Can you work these out from the model? Positions are in its coordinate system, mm. Give positions to 0.01 mm unless a question says otherwise; leave off trailing zeros. Order: outer loops, then holes, each group sorted by start corner. A loop starts at its lowest first (then second) coordinate and runs counter-clockwise, first axis right, second up. Notation, with made-up numbers: (-29.75, 72) - (-24.75, 72) arc R8 ccw to (-24.75, 80) - close; hole circle Ø6 at (78.5, 69.5). An arc over 180 degrees is marked (long way). Answer as a JSON object with one key per item and string values.
```python
from build123d import *

# Parameters (mm, degrees)
BOSS_EXTRUDE1_DEPTH  = 4.7625
M4_CLEARANCE_HOLE1_D = 4.5


with BuildPart() as part:
    # Sketch2 → Boss-Extrude1 (new body)
    with BuildSketch(Plane.XY):
        with BuildLine():
            Line((-58.18125, 21.734258268), (-58.18125, -30.061313165))
            ThreePointArc((-58.18125, -30.061313165), (-59.147979937, -34.921392756), (-61.900993879, -39.041569286))
            Line((-61.900993879, -39.041569286), (-63.182817689, -40.323393096))
            ThreePointArc((-63.182817689, -40.323393096), (-63.182817689, -48.101567689), (-55.404643096, -48.101567689))
            Line((-55.404643096, -48.101567689), (-54.122819286, -46.819743879))
            ThreePointArc((-54.122819286, -46.819743879), (-50.002642756, -44.066729937), (-45.142563165, -43.1))
            Line((-45.142563165, -43.1), (45.142563165, -43.1))
            ThreePointArc((45.142563165, -43.1), (50.002642756, -44.066729937), (54.122819286, -46.819743879))
            Line((54.122819286, -46.819743879), (55.404643096, -48.101567689))
            ThreePointArc((55.404643096, -48.101567689), (63.182817689, -48.101567689), (63.182817689, -40.323393096))
            Line((63.182817689, -40.323393096), (61.900993879, -39.041569286))
            ThreePointArc((61.900993879, -39.041569286), (59.147979937, -34.921392756), (58.18125, -30.061313165))
            Line((58.18125, -30.061313165), (58.18125, 21.734258268))
            ThreePointArc((58.18125, 21.734258268), (59.919591901, 28.147685724), (64.658738462, 32.805407718))
            ThreePointArc((64.658738462, 32.805407718), (67.284676339, 38.9927926), (61.96395, 43.1))
            Line((61.96395, 43.1), (-61.96395, 43.1))
            ThreePointArc((-61.96395, 43.1), (-67.284676339, 38.9927926), (-64.658738462, 32.805407718))
            ThreePointArc((-64.658738462, 32.805407718), (-59.919591901, 28.147685724), (-58.18125, 21.734258268))
        make_face()
    extrude(amount=BOSS_EXTRUDE1_DEPTH)

    # M4 Clearance Hole1 (through all)
    with Locations(Plane.XY.offset(4.7625)):
        with Locations((-59.293730392, -44.212480392), (-61.96395, 37.6), (61.96395, 37.6), (59.293730392, -44.212480392)):
            Hole(M4_CLEARANCE_HOLE1_D / 2)


solid = part.part
```
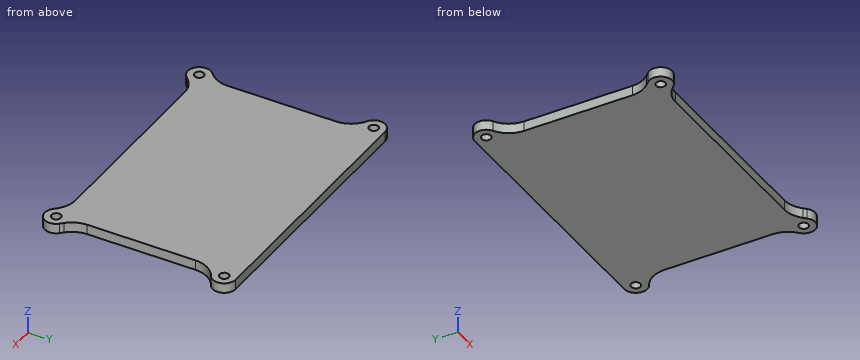
Q1. If we section it at A-A, the plane y = 37.6: Please give me the cut outline in (x, z).
Recorded:
{"outline": "(-67.46, 0) - (-64.21, 0) - (-64.21, 4.76) - (-67.46, 4.76) - close; (-59.71, 0) - (59.71, 0) - (59.71, 4.76) - (-59.71, 4.76) - close; (64.21, 0) - (67.46, 0) - (67.46, 4.76) - (64.21, 4.76) - close"}
Q2. I need wall thicknesses on L1, parallel to X at y = -10, z = 3.1; L2, parallel to Y at x = 37.5, z = 1.45; L3, parallel to Y at x = 58, z = 4.2. Which ranges of each line are inside material? Lowest first, please.
Recorded:
{"L1": "x = -58.18 to 58.18", "L2": "y = -43.1 to 43.1", "L3": "y = -49.56 to -46.05, -42.37 to 43.1"}
Q3. If we section it at C-C, the plane z = 3.1: Please give me the cut outline in (x, y).
Recorded:
{"outline": "(-64.66, 32.81) arc R12.7 cw to (-58.18, 21.73) - (-58.18, -30.06) arc R12.7 cw to (-61.9, -39.04) - (-63.18, -40.32) arc R5.5 ccw to (-55.4, -48.1) - (-54.12, -46.82) arc R12.7 cw to (-45.14, -43.1) - (45.14, -43.1) arc R12.7 cw to (54.12, -46.82) - (55.4, -48.1) arc R5.5 ccw to (63.18, -40.32) - (61.9, -39.04) arc R12.7 cw to (58.18, -30.06) - (58.18, 21.73) arc R12.7 cw to (64.66, 32.81) arc R5.5 ccw to (61.96, 43.1) - (-61.96, 43.1) arc R5.5 ccw to start; hole circle Ø4.5 at (-61.96, 37.6); hole circle Ø4.5 at (-59.29, -44.21); hole circle Ø4.5 at (59.29, -44.21); hole circle Ø4.5 at (61.96, 37.6)"}
Q4. If we section it at B-B, the plane x = -11.5: Please give me the cut outline in (y, z).
Recorded:
{"outline": "(-43.1, 0) - (43.1, 0) - (43.1, 4.76) - (-43.1, 4.76) - close"}
Q5. I'm going to push flat-ended pins straight in: pin 1 Ø2.5 at (y, z) = (1, 3.5) entering from +X; pin 2 Ø1 at (x, z) = (-18.5, 0.5) entering from -Y; pin 3 Ø1.4 at (y, z) = (-4.5, 3.5) entering from -X; pin 4 Ø2.5 at (x, y) = (59.29, -44.21) entering from -Z. Where does each tip first touch, or does it pass through?
Recorded:
{"pin 1": "stops at x = 58.18", "pin 2": "stops at y = -43.1", "pin 3": "stops at x = -58.18", "pin 4": "passes through"}
Q6. If we section it at D-D, the plane y = 11: Please give me the cut outline in (x, z).
Recorded:
{"outline": "(-58.18, 0) - (58.18, 0) - (58.18, 4.76) - (-58.18, 4.76) - close"}
